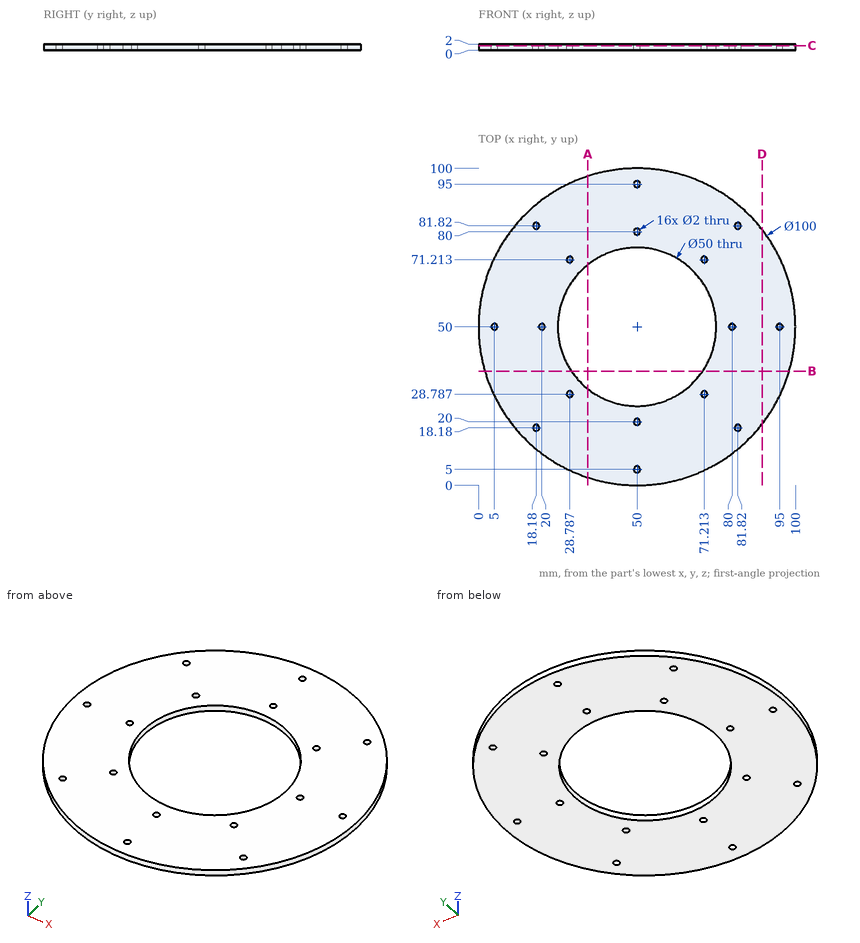
Study the drawing (mm; zero at the part's minimum x, y, z) and answer. Round coordinates to 2 decimals unless told otherwise and drop trailing zeros. Loops run counter-clockwise (first coordinate to the right, second up) from the corner with the lowest first, then second, coordinate; pieces in that order, holes last.
Q1. Section A-A, the plane x = 34.5 is taken. Determine the outline of the cut face in (y, z) (1 decimal).
Q2. Section B-B, the plane y = 36 is taken. Determine the outline of the cut face in (x, z), then the cut area to 3 significant figures.
Q3. Section D-D, the plane x = 89.5 is taken. Determine the outline of the cut face in (y, z) (1 decimal), then the cut area to 3 significant figures.
Q4. Section C-C, the plane z = 1.45 is taken. Count the separate pieces of the cut face and the enclosed holes in it, then the cut area to 3 significant figures.
Q5. Find the intervals of material crossed by line 1 (X direction, y = 29, z = 1.2) (1 decimal); line 2 (Y direction, x = 58.5, z = 1.05); line 3 (Y direction, x = 67.5, z = 1.9), in increasing order.
Q6. Given pin 1 Ø1 at (x, z) = (38, 0.5) entering from +Y; pin 2 Ø1.6 at (x, y) = (80, 50) entering from +Z, each flat-ended and moving along its own axis, determine where each tip first touches the part or whether it passes through.
Completed:
1. outline: (2.5, 0) - (30.4, 0) - (30.4, 2) - (2.5, 2) - close; (69.6, 0) - (97.5, 0) - (97.5, 2) - (69.6, 2) - close
2. outline: (2, 0) - (29.29, 0) - (29.29, 2) - (2, 2) - close; (70.71, 0) - (98, 0) - (98, 2) - (70.71, 2) - close
2. area: 109 mm2
3. outline: (19.3, 0) - (80.7, 0) - (80.7, 2) - (19.3, 2) - close
3. area: 123 mm2
4. separate pieces: 1
4. enclosed holes: 17
4. area: 5,840 mm2
5. line 1: x = 4.6 to 27.8, 29.8 to 36.4, 63.6 to 70.2, 72.2 to 95.4
5. line 2: y = 0.73 to 26.49, 73.51 to 99.27
5. line 3: y = 3.16 to 32.15, 67.85 to 96.84
6. pin 1: stops at y = 98.66
6. pin 2: passes through
